```python
from build123d import *

# Parameters (mm, degrees)
BOSS_EXTRUDE1_DEPTH = 447.04


with BuildPart() as part:
    # Sketch1 → Boss-Extrude1 (new body)
    with BuildSketch(Plane(origin=(0, 0, 0), x_dir=(1, 0, 0), z_dir=(0, 1, 0))):
        with BuildLine():
            ThreePointArc((0, 12.7), (3.719743879, 3.719743879), (12.7, 0))
            Line((12.7, 0), (12.7, 3.175))
            Line((12.7, 3.175), (19.05, 3.175))
            Line((19.05, 3.175), (19.05, 19.05))
            Line((19.05, 19.05), (3.175, 19.05))
            Line((3.175, 19.05), (3.175, 12.7))
            Line((3.175, 12.7), (0, 12.7))
        make_face()
    extrude(amount=BOSS_EXTRUDE1_DEPTH)


solid = part.part
```
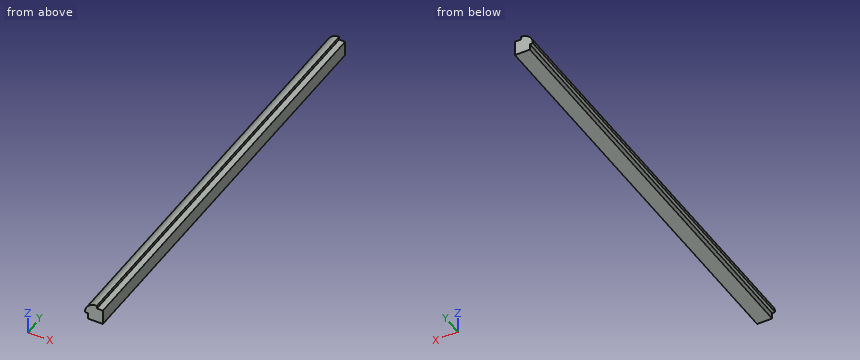
For this review, take the finished solid that the model builds, in its own axes (mm). Coordinates: 2 decimals unless noted, no trailing zeros. Write each loop counter-clockwise with the first axis right and the second up, starting at its lowest first coordinate (ties: lowest second). Pieces come first, ordered by that corner, then holes. Notation, with made-up numbers: (79, 8.25) - (109, 8.25) arc R20 cw to (109, 13.25) - close; hole circle Ø5 at (77, 7.5). An arc over 180 degrees is marked (long way). Answer in a Markdown table with one row per item. Add a question column.
Q1. We need section B-B, the plane x = 15.75. State the section outline as (y, z) points (3 decimals).
Q2. For P1, Ø8, axis at x = 12.5, z = -8, coming from the -Y side; P2, Ø3, axis at x = 17, y = 299, coming from the +Z side (3 decimals); P3, Ø2.5, axis at y = 280, z = -1, coming from the +X side; P4, Ø4, axis at y = 163.5, z = -4, coming from the -X side, all flat-tipped, find the tip position at first contact; note any pin that passes through.
Q3. We need section A-A, the plane y = 146. State the section outline as (x, z) points (3 decimals).
Q4. For probe 1 along X at (y, z) = (309.5, -11.75); probe 2 along X at (y, z) = (197.5, -15.25) (3 decimals); probe 3 along Z at (x, y) = (12.25, 229.5), list the stretches that pass through material, from the lowest coordinate up.
Q5. We need section C-C, the plane z = -9.5. State the section outline as (x, y) points.
Answer list:
| question | item | result |
|---|---|---|
| 1 | outline | (0, -19.05) - (447.04, -19.05) - (447.04, -3.175) - (0, -3.175) - close |
| 2 | P1 | stops at y = 0 |
| 2 | P2 | stops at z = -3.175 |
| 2 | P3 | stops at x = 12.7 |
| 2 | P4 | stops at x = 1.91 |
| 3 | outline | (0, -12.7) - (3.175, -12.7) - (3.175, -19.05) - (19.05, -19.05) - (19.05, -3.175) - (12.7, -3.175) - (12.7, 0) arc R12.7 ccw to start |
| 4 | probe 1 | x = 0.04 to 19.05 |
| 4 | probe 2 | x = 3.175 to 19.05 |
| 4 | probe 3 | z = -19.05 to -0.01 |
| 5 | outline | (0.41, 0) - (19.05, 0) - (19.05, 447.04) - (0.41, 447.04) - close |
